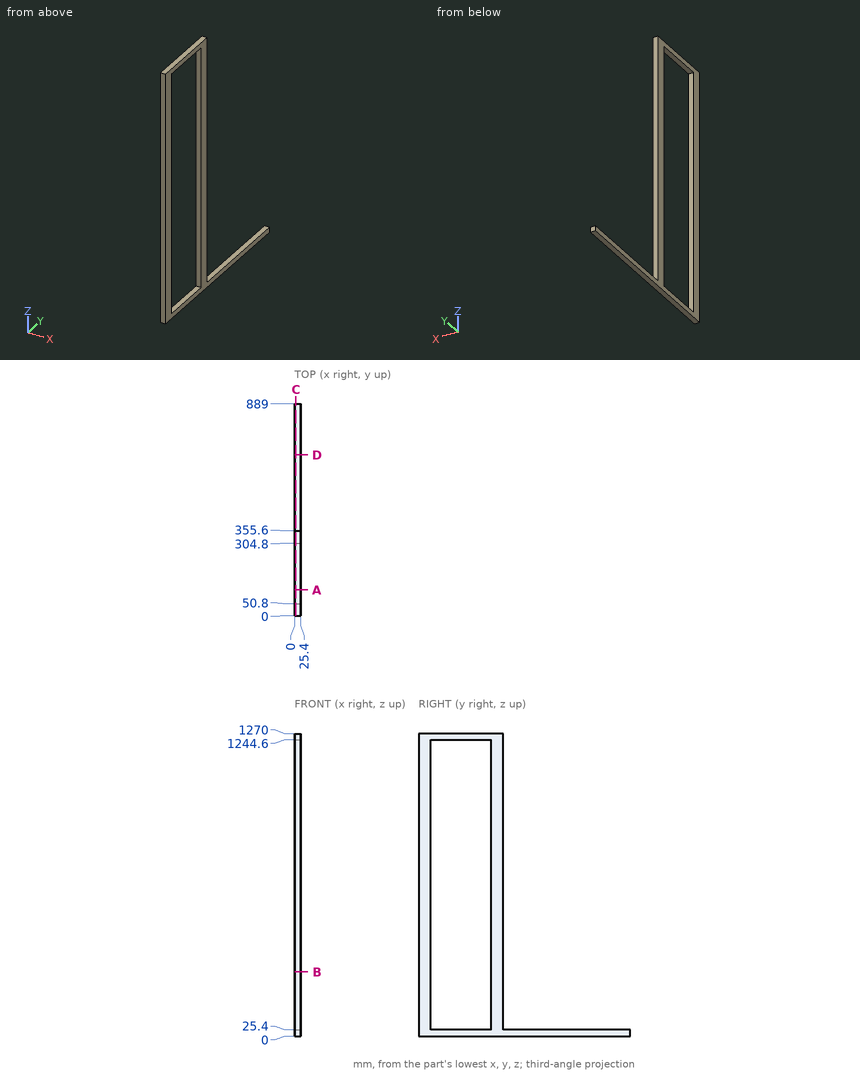
Geometry: see drawing. Coordinates: mm, zero at the bounding-box minimum. Round coordinates to 2 decimals unless told otherwise and drop trailing zeros. Write each loop counter-clockwise with the first axis right and the second up, starting at its lowest first coordinate (ties: lowest second). Pieces come first, ordered by that corner, then holes.
Item 1: Pin query (flat end, axial travel): P1, Ø7.5, axis at x = 13, z = 398, coming from the +Y side; P2, Ø7.5, axis at x = 7.5, y = 490.5, coming from the +Z side. Return the tip coordinate at first contact, or that it passes through.
Item 2: Section query C-C (x = 5.25). Return loops of the section in (y, z), plus the area to 3 significant figures.
Item 3: Section query A-A (y = 108). Return loops of the section in (x, z), plus the area to 3 significant figures.
Item 4: Section query D-D (y = 675). Return loops of the section in (x, z), plus the area to 3 significant figures.
Item 5: Material intervals for L1, parallel to Y at x = 10, z = 442; L2, parallel to Z at x = 9.25, y = 268; L3, parallel to Z at x = 13.25, y = 407, sorted ascending.
Item 6: Section query B-B (z = 269.5). Return loops of the section in (x, y).
Completed:
1. P1: stops at y = 355.6
1. P2: stops at z = 25.4
2. outline: (0, 0) - (889, 0) - (889, 25.4) - (355.6, 25.4) - (355.6, 1270) - (0, 1270) - close; hole (50.8, 25.4) - (304.8, 25.4) - (304.8, 1244.6) - (50.8, 1244.6) - close
2. area: 155,000 mm2
3. outline: (0, 0) - (25.4, 0) - (25.4, 25.4) - (0, 25.4) - close; (0, 1244.6) - (25.4, 1244.6) - (25.4, 1270) - (0, 1270) - close
3. area: 1,290 mm2
4. outline: (0, 0) - (25.4, 0) - (25.4, 25.4) - (0, 25.4) - close
4. area: 645 mm2
5. L1: y = 0 to 50.8, 304.8 to 355.6
5. L2: z = 0 to 25.4, 1244.6 to 1270
5. L3: z = 0 to 25.4
6. outline: (0, 0) - (25.4, 0) - (25.4, 50.8) - (0, 50.8) - close; (0, 304.8) - (25.4, 304.8) - (25.4, 355.6) - (0, 355.6) - close
